from build123d import *

# Parameters (mm, degrees)
SKETCH_1_W          = 32
SKETCH_1_H          = 20
EXTRUDE_1_DEPTH     = 6
SKETCH_2_W          = 32
SKETCH_2_H          = 6
EXTRUDE_2_DEPTH     = 55
SKETCH_3_R          = 17
CUT_EXTRUDE_1_DEPTH = 55


with BuildPart() as part:
    # 草图1 → 凸台-拉伸1 (new body)
    with BuildSketch(Plane(origin=(0, 0, 0), x_dir=(1, 0, 0), z_dir=(0, 1, 0))):
        with Locations((0, 11.560693642)):
            Rectangle(SKETCH_1_W, SKETCH_1_H)
    extrude(amount=EXTRUDE_1_DEPTH)

    # 草图2 → 凸台-拉伸2 (add)
    with BuildSketch(Plane(origin=(0, 6, 0), x_dir=(1, 0, 0), z_dir=(0, 1, 0))):
        with Locations((0, 4.560693642)):
            Rectangle(SKETCH_2_W, SKETCH_2_H)
    extrude(amount=EXTRUDE_2_DEPTH)

    # 草图3 → 切除-拉伸1 (cut)
    with BuildSketch(Plane.XY.offset(-1.560693642)):
        with Locations((0, 73)):
            Circle(SKETCH_3_R)
    extrude(amount=-CUT_EXTRUDE_1_DEPTH, mode=Mode.SUBTRACT)


solid = part.part
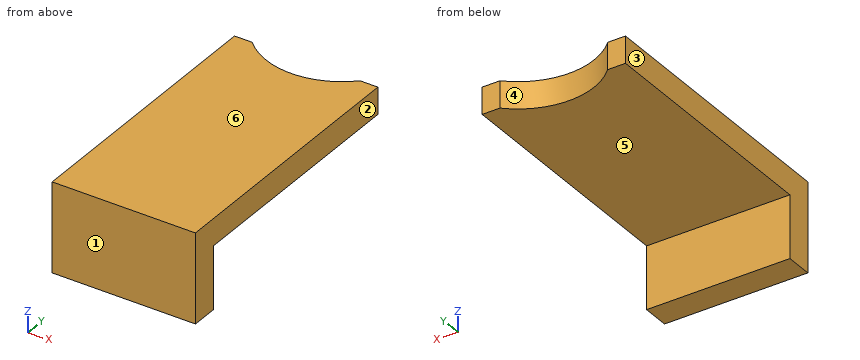
CAD build for the part. Positions are in the model's coordinates, mm. Face numbers are marked on the shaded views. A direction names the side the tool comes from. Coordinates: 2 decimals unless noted, no trailing zeros. Write each loop counter-clockwise with the first axis right and the second up, starting at its lowest first coordinate (ties: lowest second). Pieces come first, ordered by that corner, then holes. Notation, with made-up numbers: (-38, 80) - (7, 80) arc R19 ccw to (7, 87) - close; hole circle Ø4 at (14.25, -21). An arc over 180 degrees is marked (long way). Use a Markdown table: item, result. Add a question column.
Item 1: Mould opens along X. For the marked faces 1, 2, 3 and 4 say: pulls with the +X half, pulls with the -X half, needs draft (parallel to the pull), parting line crosses it, or undercut.
Item 2: 3-axis set-ups, long thin cutter, end or side, ignore diameter. For the marked faces 5 and 6: which of +Z, -Z, +X, -X, +Y, -Y reach the whole face in a straight line?
Item 3: Drill centre lines: L1, parallel to Z at x = -11, y = 36; L2, parallel to Y at x = -14, z = -20; L3, parallel to Y at x = 8.5, z = -4.25. Where is each one in solid material? Low to high. Write a range as from..to.
Item 4: Band-saw the part on D-D, the plane z = -15.25. Give the cut face in (x, y), and give its area (3 significant figures).
Item 5: Band-saw the part on C-C, the plane y = 43. Give the cut face in (x, z).
Item 6: Band-saw the part on A-A, the plane x = -13. Give the cut face in (y, z), and give its area (3 significant figures).
Item 7: Band-saw the part on B-B, the plane z = -3. Give the cut face in (x, y).
Item 8: Flat gauge pins, fed straight in: pin 1 (11 mm diameter, centred on x = -5.5, z = -15.5, fed in from +Y); pin 2 (1.5 mm diameter, centred on x = -11.5, y = 48, fed in from -Z). Where does each tip first touch, or does it go through?
Numbers:
| question | item | result |
|---|---|---|
| 1 | face 1 | needs draft |
| 1 | face 2 | pulls with the +X half |
| 1 | face 3 | pulls with the -X half |
| 1 | face 4 | undercut |
| 2 | face 5 | -Z, +X, -X, +Y |
| 2 | face 6 | +Z, +X, -X, +Y, -Y |
| 3 | L1 | -7.56..-1.56 |
| 3 | L2 | 0..6 |
| 3 | L3 | 0..58.28 |
| 4 | outline | (-16, 0) - (16, 0) - (16, 6) - (-16, 6) - close |
| 4 | area | 192 mm2 |
| 5 | outline | (-16, -7.56) - (16, -7.56) - (16, -1.56) - (-16, -1.56) - close |
| 6 | outline | (0, -21.56) - (6, -21.56) - (6, -7.56) - (61, -7.56) - (61, -1.56) - (0, -1.56) - close |
| 6 | area | 450 mm2 |
| 7 | outline | (-16, 0) - (16, 0) - (16, 61) - (12.04, 61) arc R17 cw to (-12.04, 61) - (-16, 61) - close |
| 8 | pin 1 | y = 6 |
| 8 | pin 2 | z = -7.56 |
